The model under review builds one solid part; all positions refer to its coordinate system, in mm. Round coordinates to 2 decimals unless told otherwise and drop trailing zeros. Loops run counter-clockwise (first coordinate to the right, second up) from the corner with the lowest first, then second, coordinate; pieces in that order, holes last. Notation, with made-up numbers: M 55,43 L 91,43 A29 cw 91,77 Z; hole C 74.5,51 d11. An arc over 180 degrees is marked long. Answer as a JSON object with one key per item and string values. Group by question number.
Item 1: Consider section B-B (y = 16.5). Give the boundary of the cut face in (x, z).
Item 2: Consider section D-D (y = -6.5). Give the boundary of the cut face in (x, z).
Item 3: Insertion check: P1, Ø3, axis at x = -34.5, z = 4, coming from the +Y side; P2, Ø10.5, axis at x = -19.5, y = -11.5, coming from the +Z side; P3, Ø4, axis at x = 11, y = -4.5, coming from the +Z side. Each pin has a flat end and moves straight along its axis. Give the tip position at first contact, or say it passes through.
Item 4: Consider section C-C (y = -14.5). Give the boundary of the cut face in (x, z), and give its area (3 significant figures).
Item 5: To check wall thickness, follow line 1 (Y direction, x = 48.5, z = -0.3); line 2 (Y direction, x = 0, z = -1); line 3 (Z direction, x = -15.5, y = -4.5). State the ranges of each line that lie inside material, in increasing order.
Item 6: Consider section A-A (x = 13). Give the boundary of the cut face in (y, z), and give its area (3 significant figures).
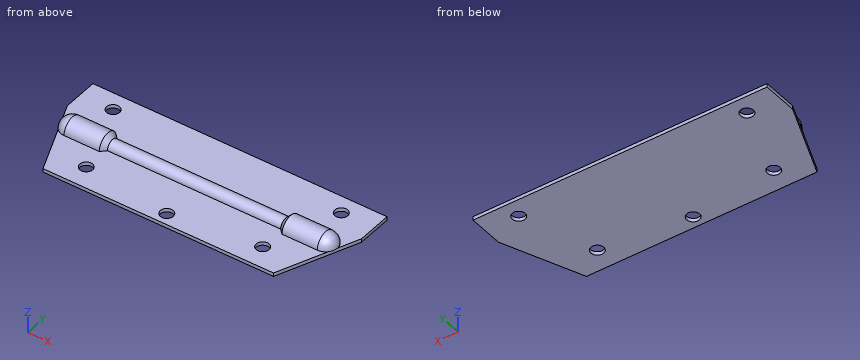
```python
from build123d import *

# Parameters (mm, degrees)
SKETCH_R         = 2.75
PAD_DEPTH        = 1.5
REVOLUTION_ANGLE = 180


with BuildPart() as part:
    # Sketch → Pad (new body)
    with BuildSketch(Plane.XY):
        Polygon((-62.5, 24), (62.5, 24), (62.5, 9), (49, -24), (-49, -24), (-62.5, 9), align=None)
        with Locations((0, -19)):
            Circle(SKETCH_R, mode=Mode.SUBTRACT)
        with Locations((37.5, -14.5)):
            Circle(SKETCH_R, mode=Mode.SUBTRACT)
        with Locations((-37.5, -14.5)):
            Circle(SKETCH_R, mode=Mode.SUBTRACT)
        with Locations((-48.5, 16.5)):
            Circle(SKETCH_R, mode=Mode.SUBTRACT)
        with Locations((48.5, 16.5)):
            Circle(SKETCH_R, mode=Mode.SUBTRACT)
    extrude(amount=-PAD_DEPTH)

    # Sketch001 → Revolution (revolve)
    with BuildSketch(Plane.XY):
        with BuildLine():
            Line((-53.818182, 5), (-38.818182, 5))
            Line((-38.818182, 5), (-36.818182, 3))
            Line((-36.818182, 3), (36.818182, 3))
            Line((36.818182, 3), (38.818182, 5))
            Line((38.818182, 5), (53.818182, 5))
            ThreePointArc((58.818182, 0), (57.353716, 3.535534), (53.818182, 5))
            Line((57.818182, 0), (58.818182, 0))
            ThreePointArc((57.818182, 0), (56.646609, 2.828427), (53.818182, 4))
            Line((53.818182, 4), (39.232395, 4))
            Line((39.232395, 4), (37.232395, 2))
            Line((37.232395, 2), (-37.232395, 2))
            Line((-37.232395, 2), (-39.232395, 4))
            Line((-39.232395, 4), (-53.818182, 4))
            ThreePointArc((-53.818182, 4), (-56.646609, 2.828427), (-57.818182, 0))
            Line((-58.818182, 0), (-57.818182, 0))
            ThreePointArc((-53.818182, 5), (-57.353716, 3.535534), (-58.818182, 0))
        make_face()
    revolve(axis=Axis((0, 0, 0), (1, 0, 0)), revolution_arc=REVOLUTION_ANGLE)


solid = part.part
```
Geometry results:
{
 "1": {"outline": "M -62.5,-1.5 L -51.25,-1.5 L -51.25,0 L -62.5,0 Z; M -45.75,-1.5 L 45.75,-1.5 L 45.75,0 L -45.75,0 Z; M 51.25,-1.5 L 62.5,-1.5 L 62.5,0 L 51.25,0 Z"},
 "2": {"outline": "M -56.16,-1.5 L 56.16,-1.5 L 56.16,0 L -56.16,0 Z"},
 "3": {"P1": "stops at y = 1.66", "P2": "stops at z = 0", "P3": "stops at z = 1.66"},
 "4": {"outline": "M -52.89,-1.5 L -40.25,-1.5 L -40.25,0 L -52.89,0 Z; M -34.75,-1.5 L 34.75,-1.5 L 34.75,0 L -34.75,0 Z; M 40.25,-1.5 L 52.89,-1.5 L 52.89,0 L 40.25,0 Z", "area": "142 mm^2"},
 "5": {"line 1": "y = -24 to 13.75, 19.25 to 24", "line 2": "y = -24 to -21.75, -16.25 to 24", "line 3": "z = -1.5 to 0"},
 "6": {"outline": "M -24,-1.5 L 24,-1.5 L 24,0 L 3,0 A3 ccw -3,0 L -24,0 Z; hole M -2,0 L 2,0 A2 ccw Z", "area": "79.9 mm^2"}
}
